```python
from build123d import *

# Parameters (mm, degrees)
SKETCH1_W           = 80
SKETCH1_H           = 25
BOSS_EXTRUDE1_DEPTH = 10
SKETCH3_2_W         = 10
SKETCH3_2_H         = 10
CUT_EXTRUDE1_DEPTH  = 7
SKETCH3_3_W         = 10
SKETCH3_3_H         = 10
CUT_EXTRUDE2_DEPTH  = 7
SKETCH3_W           = 10
SKETCH3_H           = 10
CUT_EXTRUDE3_DEPTH  = 7
SKETCH3_6_W         = 10
SKETCH3_6_H         = 10
CUT_EXTRUDE4_DEPTH  = 7
SKETCH3_7_W         = 10
SKETCH3_7_H         = 10
CUT_EXTRUDE5_DEPTH  = 7
SKETCH3_8_W         = 10
SKETCH3_8_H         = 10
CUT_EXTRUDE6_DEPTH  = 7
SKETCH3_9_W         = 10
SKETCH3_9_H         = 10
CUT_EXTRUDE7_DEPTH  = 7
SKETCH3_10_W        = 10
SKETCH3_10_H        = 10
CUT_EXTRUDE8_DEPTH  = 7
SKETCH3_11_W        = 10
SKETCH3_11_H        = 10
CUT_EXTRUDE9_DEPTH  = 7
SKETCH3_12_W        = 10
SKETCH3_12_H        = 10
CUT_EXTRUDE10_DEPTH = 7
SKETCH4_W           = 16.29
SKETCH4_H           = 25
BOSS_EXTRUDE2_DEPTH = 10
SKETCH5_W           = 10
SKETCH5_H           = 10
CUT_EXTRUDE12_DEPTH = 7
SKETCH6_W           = 6.292169455
SKETCH6_H           = 25
SKETCH6_W_2         = 6.29
BOSS_EXTRUDE3_DEPTH = 3


with BuildPart() as part:
    # Sketch1 → Boss-Extrude1 (new body)
    with BuildSketch(Plane.XY):
        with Locations((40, -12.5)):
            Rectangle(SKETCH1_W, SKETCH1_H)
    extrude(amount=BOSS_EXTRUDE1_DEPTH)

    # Sketch3<2> → Cut-Extrude1 (cut)
    with BuildSketch(Plane.XY.offset(10)):
        with Locations((11.292169455, -5)):
            Rectangle(SKETCH3_2_W, SKETCH3_2_H)
    extrude(amount=-CUT_EXTRUDE1_DEPTH, mode=Mode.SUBTRACT)

    # Sketch3<3> → Cut-Extrude2 (cut)
    with BuildSketch(Plane.XY.offset(10)):
        with Locations((25.292169455, -5)):
            Rectangle(SKETCH3_3_W, SKETCH3_3_H)
    extrude(amount=-CUT_EXTRUDE2_DEPTH, mode=Mode.SUBTRACT)

    # Sketch3 → Cut-Extrude3 (cut)
    with BuildSketch(Plane.XY.offset(10)):
        with Locations((39.292169455, -5)):
            Rectangle(SKETCH3_W, SKETCH3_H)
    extrude(amount=-CUT_EXTRUDE3_DEPTH, mode=Mode.SUBTRACT)

    # Sketch3<6> → Cut-Extrude4 (cut)
    with BuildSketch(Plane.XY.offset(10)):
        with Locations((53.292169455, -5)):
            Rectangle(SKETCH3_6_W, SKETCH3_6_H)
    extrude(amount=-CUT_EXTRUDE4_DEPTH, mode=Mode.SUBTRACT)

    # Sketch3<7> → Cut-Extrude5 (cut)
    with BuildSketch(Plane.XY.offset(10)):
        with Locations((67.292169455, -5)):
            Rectangle(SKETCH3_7_W, SKETCH3_7_H)
    extrude(amount=-CUT_EXTRUDE5_DEPTH, mode=Mode.SUBTRACT)

    # Sketch3<8> → Cut-Extrude6 (cut)
    with BuildSketch(Plane.XY.offset(10)):
        with Locations((67.292169455, -20)):
            Rectangle(SKETCH3_8_W, SKETCH3_8_H)
    extrude(amount=-CUT_EXTRUDE6_DEPTH, mode=Mode.SUBTRACT)

    # Sketch3<9> → Cut-Extrude7 (cut)
    with BuildSketch(Plane.XY.offset(10)):
        with Locations((53.292169455, -20)):
            Rectangle(SKETCH3_9_W, SKETCH3_9_H)
    extrude(amount=-CUT_EXTRUDE7_DEPTH, mode=Mode.SUBTRACT)

    # Sketch3<10> → Cut-Extrude8 (cut)
    with BuildSketch(Plane.XY.offset(10)):
        with Locations((39.292169455, -20)):
            Rectangle(SKETCH3_10_W, SKETCH3_10_H)
    extrude(amount=-CUT_EXTRUDE8_DEPTH, mode=Mode.SUBTRACT)

    # Sketch3<11> → Cut-Extrude9 (cut)
    with BuildSketch(Plane.XY.offset(10)):
        with Locations((25.292169455, -20)):
            Rectangle(SKETCH3_11_W, SKETCH3_11_H)
    extrude(amount=-CUT_EXTRUDE9_DEPTH, mode=Mode.SUBTRACT)

    # Sketch3<12> → Cut-Extrude10 (cut)
    with BuildSketch(Plane.XY.offset(10)):
        with Locations((11.292169455, -20)):
            Rectangle(SKETCH3_12_W, SKETCH3_12_H)
    extrude(amount=-CUT_EXTRUDE10_DEPTH, mode=Mode.SUBTRACT)

    # Sketch4 → Boss-Extrude2 (add)
    with BuildSketch(Plane.XY.offset(10)):
        with Locations((84.437169455, -12.5)):
            Rectangle(SKETCH4_W, SKETCH4_H)
    extrude(amount=-BOSS_EXTRUDE2_DEPTH)

    # Sketch5 → Cut-Extrude12 (cut)
    with BuildSketch(Plane.XY.offset(10)):
        with Locations((81.292169455, -5)):
            Rectangle(SKETCH5_W, SKETCH5_H)
        with Locations((81.292169455, -20)):
            Rectangle(SKETCH5_W, SKETCH5_H)
    extrude(amount=-CUT_EXTRUDE12_DEPTH, mode=Mode.SUBTRACT)

    # Sketch6 → Boss-Extrude3 (add)
    with BuildSketch(Plane.XY.offset(10)):
        with Locations((3.146084728, -12.5)):
            Rectangle(SKETCH6_W, SKETCH6_H)
        with Locations((89.437169455, -12.5)):
            Rectangle(SKETCH6_W_2, SKETCH6_H)
    extrude(amount=BOSS_EXTRUDE3_DEPTH)


solid = part.part
```
Could you check a few things on this model? Use its own coordinates, in mm. A direction names the side the tool comes from. Give positions to 0.01 mm unless a question says otherwise; leave off trailing zeros. Write each loop counter-clockwise with the first axis right and the second up, starting at its lowest first coordinate (ties: lowest second). Pieces come first, ordered by that corner, then holes. Notation, with made-up numbers: (58.5, 7) - (109.5, 7) arc R25 cw to (109.5, 46) - close; hole circle Ø7 at (61.25, -22). An arc over 180 degrees is marked (long way). One line per item, written item: value. Start each with the question number.
Item 1: Imagine slicing it at B-B, the plane x = 80. List the corners of the cut face in (y, z) for me.
Item 2: Imagine slicing it at C-C, the plane y = -12.5. List the corners of the cut face in (x, z) for me.
Item 3: I'm going to push flat-ended pins straight in: pin 1 (4 mm diameter, centred on x = 65.5, y = -17.5, fed in from +Z); pin 2 (8 mm diameter, centred on x = 69.5, y = -5, fed in from +Z); pin 3 (2 mm diameter, centred on x = 54.5, z = 6.5, fed in from +Y). Where does each tip first touch, or does it pass through?
Item 4: Which directions (+Z, -Z, +X, -X, +Y, -Y) give clear straight access to the entire face, cutting with the end or side of a thin tool? Please do faces 1 (the face through (46, -25, 5)), 2 (the face through (67, -20, 3)), 3 (the face through (76.292, -5, 7)).
Item 5: Please list where these lines run through material, in increasing order: line 1 (X direction, y = -1.75, z = 11.5); line 2 (Z direction, x = 28, y = -23); line 3 (Y direction, x = 68.5, z = 7.25). Write a range as from..to.
Item 6: Imagine slicing it at A-A, the plane y = -22.75. List the corners of the cut face in (x, z) for me, and give its area (3 significant figures).
Item 7: Imagine slicing it at D-D, the plane x = 45.5. List the corners of the cut face in (y, z) for me, and give its area (3 significant figures).
Geometry says:
1. outline: (-25, 0) - (0, 0) - (0, 3) - (-10, 3) - (-10, 10) - (-15, 10) - (-15, 3) - (-25, 3) - close
2. outline: (0, 0) - (92.58, 0) - (92.58, 13) - (86.29, 13) - (86.29, 10) - (6.29, 10) - (6.29, 13) - (0, 13) - close
3. pin 1: z = 3
3. pin 2: z = 10
3. pin 3: y = -10
4. face 1: +Z, -Z, +X, -X, -Y
4. face 2: +Z, -Y
4. face 3: +Z, +Y
5. line 1: 0..6.29, 86.29..92.58
5. line 2: 0..3
5. line 3: -15..-10
6. outline: (0, 0) - (92.58, 0) - (92.58, 13) - (86.29, 13) - (86.29, 3) - (76.29, 3) - (76.29, 10) - (72.29, 10) - (72.29, 3) - (62.29, 3) - (62.29, 10) - (58.29, 10) - (58.29, 3) - (48.29, 3) - (48.29, 10) - (44.29, 10) - (44.29, 3) - (34.29, 3) - (34.29, 10) - (30.29, 10) - (30.29, 3) - (20.29, 3) - (20.29, 10) - (16.29, 10) - (16.29, 3) - (6.29, 3) - (6.29, 13) - (0, 13) - close
6. area: 544 mm^2
7. outline: (-25, 0) - (0, 0) - (0, 10) - (-25, 10) - close
7. area: 250 mm^2
